CAD build for the part. Positions are in the model's coordinates, mm. A direction names the side the tool comes from. Round coordinates to 2 decimals unless told otherwise and drop trailing zeros. Loops run counter-clockwise (first coordinate to the right, second up) from the corner with the lowest first, then second, coordinate; pieces in that order, holes last. Notation, with made-up numbers: (59.5, -38) -> (90.5, -38) arc R17 cw to (90.5, -12) -> close; hole circle Ø9 at (5.25, 31). An arc over 180 degrees is marked (long way). Answer as CSV lines item,"result".
```python
from build123d import *

# Parameters (mm, degrees)
EXTRUDE_1_DEPTH          = 6
CUT_EXTRUDE_1_DEPTH      = 35.74465435
CUT_EXTRUDE_1_DEPTH_BACK = 35.74465435
SKETCH_2_R               = 1.7


with BuildPart() as part:
    # 草图1 → 凸台-拉伸1 (new body)
    with BuildSketch(Plane.XY):
        with BuildLine():
            Line((20.071646816, 19.6), (-12.15, 19.6))
            ThreePointArc((-12.15, 19.6), (-18.761448404, 16.861448404), (-21.5, 10.25))
            Line((-21.5, 10.25), (-21.5, -10.25))
            ThreePointArc((-21.5, -10.25), (-18.761448404, -16.861448404), (-12.15, -19.6))
            Line((-12.15, -19.6), (20.071646816, -19.6))
            ThreePointArc((20.071646816, -19.6), (28.054072893, 0), (20.071646816, 19.6))
        make_face()
        with BuildLine():
            ThreePointArc((11.6217341, 13.850243366), (15.167616283, 15.432881266), (18.601156804, 13.619370123))
            ThreePointArc((18.601156804, 13.619370123), (23.054072893, 0), (18.601156804, -13.619370123))
            ThreePointArc((18.601156804, -13.619370123), (15.167616283, -15.432881266), (11.6217341, -13.850243366))
            Line((11.6217341, -13.850243366), (-12.15, -13.850243366))
            ThreePointArc((-12.15, -13.850243366), (-15.750243366, -10.25), (-12.15, -6.649756634))
            Line((-12.15, -6.649756634), (-8.3, -6.649756634))
            Line((-8.3, -6.649756634), (-8.3, -3.649756634))
            Line((-8.3, -3.649756634), (-12.15, -3.649756634))
            ThreePointArc((-12.15, -3.649756634), (-14.695756498, -2.595269766), (-15.750243366, -0.049513268))
            Line((-15.750243366, -0.049513268), (-15.750243366, 0.049513268))
            ThreePointArc((-15.750243366, 0.049513268), (-14.695756498, 2.595269766), (-12.15, 3.649756634))
            Line((-12.15, 3.649756634), (-8.3, 3.649756634))
            Line((-8.3, 3.649756634), (-8.3, 6.649756634))
            Line((-8.3, 6.649756634), (-12.15, 6.649756634))
            ThreePointArc((-12.15, 6.649756634), (-15.750243366, 10.25), (-12.15, 13.850243366))
            Line((-12.15, 13.850243366), (11.6217341, 13.850243366))
        make_face(mode=Mode.SUBTRACT)
    extrude(amount=EXTRUDE_1_DEPTH)

    # 草图2 → 切除-拉伸1 (cut, two sides: drawn at the far end of the back side and taken through both)
    with BuildSketch(Plane(origin=(0, 0, 0), x_dir=(0, 0, -1), z_dir=(1, 0, 0)).offset(-CUT_EXTRUDE_1_DEPTH_BACK)):
        with Locations((-3, -0.049513268)):
            Circle(SKETCH_2_R)
    extrude(amount=CUT_EXTRUDE_1_DEPTH + CUT_EXTRUDE_1_DEPTH_BACK, mode=Mode.SUBTRACT)


solid = part.part
```
Q1. Tool access for faces 4 (the cylindrical face through (-18.83, -16.79, 2.96)), 5 (the cylindrical face through (15.22, -15.43, 2.96)): list every direction of +Z, -Z, +X, -X, +Y, -Y with a clear straight run to the whole face (end or side of a thin tool).
Results:
face 4,"+Z, -Z, -X, -Y"
face 5,"+Z, -Z"
Q2. Slice it at B-B, the plane z = 2.75. Give the cut face in (x, y).
Results:
outline,"(-21.5, -10.25) arc R9.35 ccw to (-12.15, -19.6) -> (20.07, -19.6) arc R28.05 ccw to (28, -1.73) -> (22.99, -1.73) arc R23.05 cw to (18.6, -13.62) arc R4.44 cw to (11.62, -13.85) -> (-12.15, -13.85) arc R3.6 cw to (-12.15, -6.65) -> (-8.3, -6.65) -> (-8.3, -3.65) -> (-12.15, -3.65) arc R3.6 cw to (-15.33, -1.73) -> (-21.5, -1.73) -> close; (-21.5, 1.63) -> (-15.38, 1.63) arc R3.6 cw to (-12.15, 3.65) -> (-8.3, 3.65) -> (-8.3, 6.65) -> (-12.15, 6.65) arc R3.6 cw to (-12.15, 13.85) -> (11.62, 13.85) arc R4.44 cw to (18.6, 13.62) arc R23.05 cw to (23, 1.63) -> (28.01, 1.63) arc R28.05 ccw to (20.07, 19.6) -> (-12.15, 19.6) arc R9.35 ccw to (-21.5, 10.25) -> close"
Q3. Drop flat-ended pins along their axis: pin 1 Ø0.9 at (y, z) = (5.5, 3) entering from +X; pin 2 Ø2 at (y, z) = (11.5, 4.5) entering from +X (3 decimals); pin 3 Ø12 at (x, y) = (12.5, 4.5) entering from +Z (3 decimals); pin 4 Ø2.5 at (y, z) = (-5.5, 2.5) entering from +X. Give the stop position or say it passes through.
Results:
pin 1,"x = 27.6"
pin 2,"x = 26.015"
pin 3,"through"
pin 4,"x = 27.73"
Q4. Two-plate mould, pull along X, no slides. Class faces 1 (the flat face through (-10, 6.65, 3)), 2 (the flat face through (4, 19.6, 3)), 3 (the cylindrical face through (28.052, -0.304, 0.958)): pulls with the +X half, pulls with the -X half, needs draft (parallel to the pull), parting line crosses it, or undercut.
Results:
face 1,"undercut"
face 2,"needs draft"
face 3,"pulls with the +X half"
Q5. Probe L1, parallel to Y at x = -9.5, z = 3.25; L2, parallel to Y at x = 1, z = 1; L3, parallel to Y at x = 24.6, z = 3. List the from-to ranges inside material, lowest first. Write a range as [from, to].
Results:
L1,"[-19.6, -13.85], [-6.65, -3.65], [3.65, 6.65], [13.85, 19.6]"
L2,"[-19.6, -13.85], [13.85, 19.6]"
L3,"[-13.49, -1.75], [1.65, 13.49]"
Q6. Slice it at C-C, the plane y = 12. Give the cut face in (x, z).
Results:
outline,"(-21.33, 0) -> (-15.3, 0) -> (-15.3, 6) -> (-21.33, 6) -> close; (19.68, 0) -> (25.36, 0) -> (25.36, 6) -> (19.68, 6) -> close"
Q7. Slice it at A-A, the plane x = -7.5. Give the cut face in (y, z), and give its area (3 significant figures).
Results:
outline,"(-19.6, 0) -> (-13.85, 0) -> (-13.85, 6) -> (-19.6, 6) -> close; (13.85, 0) -> (19.6, 0) -> (19.6, 6) -> (13.85, 6) -> close"
area,"69.0 mm2"
